Read the model definition and answer for the solid it produces. Units are mm, in the model's axes. Face numbers are marked on the shaded views. A direction names the side the tool comes from. Give positions to 0.01 mm unless a question says otherwise; leave off trailing zeros. Loops run counter-clockwise (first coordinate to the right, second up) from the corner with the lowest first, then second, coordinate; pieces in that order, holes last. Notation, with made-up numbers: (0.5, 80) - (5.5, 80) arc R27 ccw to (5.5, 110) - close; hole circle Ø4 at (74.5, 69). An arc over 180 degrees is marked (long way). Write item = value, one per line.
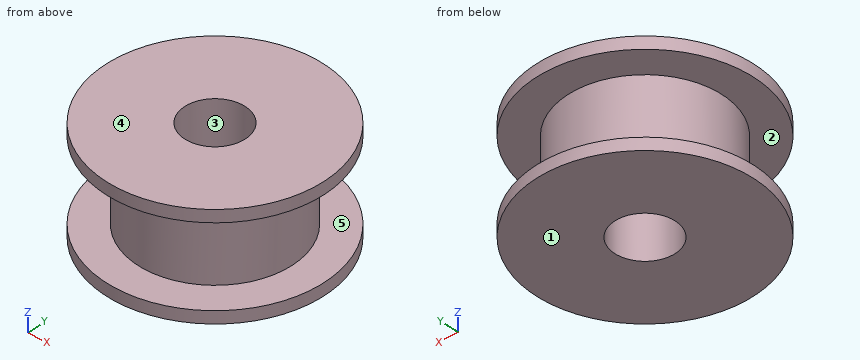
Autodesk Inventor part; units mm, degrees
ref_plane "YZ Plane" through (0, 0, 0) normal (1, 0, 0) x (0, 1, 0)
ref_plane "XZ Plane" through (0, 0, 0) normal (0, 1, 0) x (-1, 0, 0)
ref_plane "XY Plane" through (0, 0, 0) normal (0, 0, 1) x (1, 0, 0)
sketch "Sketch1" plane through (0, 0, 0) normal (0, 0, 1) x (1, 0, 0)
  circle A0 centre (0, 0) radius 6.3662
  dimension "d0" = 12.7324
extrude "Extrusion1" add sketch "Sketch1" along normal blind 8.6
sketch "Sketch2" plane through (0, 0, 8.6) normal (0, 0, 1) x (1, 0, 0)
  circle A0 centre (0, 0) radius 6.3662
  circle A1 centre (0, 0) radius 9
  dimension "d5" = 18
extrude "Extrusion2" add sketch "Sketch2" against normal blind 1
sketch "Sketch3" plane through (0, 0, 0) normal (0, 0, -1) x (-1, 0, 0)
  circle A0 centre (0, 0) radius 6.3662
  circle A1 centre (0, 0) radius 6.3662
  circle A2 centre (0, 0) radius 9
extrude "Extrusion3" add sketch "Sketch3" against normal blind 1
sketch "Sketch4" plane through (0, 0, 0) normal (0, 0, -1) x (-1, 0, 0)
  circle A0 centre (0, 0) radius 9
  circle A1 centre (0, 0) radius 2.5
  dimension "d11" = 5
extrude "Extrusion4" cut sketch "Sketch4" against normal through all contours A1
properties part number "idler"
1) A tool of negligible diameter and unlimited length cuts with its end or side. For the marked faces 1 and 2, from which of +Z, -Z, +X, -X, +Y, -Y can it reach the whole face along a straight path? Write none if from no direction.
Output:
face_1 = -Z, +X, -X, +Y, -Y
face_2 = none
2) The mould has two halves that part along Z. Classify the marked faces 3, 4 and 5: pulls with the +Z half, pulls with the -Z half, needs draft (parallel to the pull), parting line crosses it, or undercut.
Output:
face_3 = needs draft
face_4 = pulls with the +Z half
face_5 = undercut
3) A cutting plane is placed at C-C on y = -3.75. Determine the outline of the cut face in (x, z).
Output:
outline = (-8.18, 0) - (8.18, 0) - (8.18, 1) - (5.14, 1) - (5.14, 7.6) - (8.18, 7.6) - (8.18, 8.6) - (-8.18, 8.6) - (-8.18, 7.6) - (-5.14, 7.6) - (-5.14, 1) - (-8.18, 1) - close
4) A cutting plane is placed at D-D on z = 4. Determine the outline of the cut face in (x, y), then the cut area to 3 significant figures.
Output:
outline = circle Ø12.73 at (0, 0); hole circle Ø5 at (0, 0)
area = 108 mm²
5) A cutting plane is placed at A-A on y = 0. Determine the outline of the cut face in (x, z).
Output:
outline = (-9, 0) - (-2.5, 0) - (-2.5, 8.6) - (-9, 8.6) - (-9, 7.6) - (-6.37, 7.6) - (-6.37, 1) - (-9, 1) - close; (2.5, 0) - (9, 0) - (9, 1) - (6.37, 1) - (6.37, 7.6) - (9, 7.6) - (9, 8.6) - (2.5, 8.6) - close
6) Find the intervals of material crossed by probe 1 along Z at (x, y) = (-6.5, 4.5); probe 2 along Y at (x, z) = (0, 2); probe 3 along Y at (x, z) = (-1, 6), in increasing order.
Output:
probe_1 = 0 to 1, 7.6 to 8.6
probe_2 = -6.37 to -2.5, 2.5 to 6.37
probe_3 = -6.29 to -2.29, 2.29 to 6.29
7) Each of these flat-tipped pins is pushed along its axis until it touches: P1, Ø5, axis at y = -4, z = 6, coming from the +X side; P2, Ø1, axis at y = -3.5, z = 6, coming from the +X side (3 decimals); P3, Ø1.5, axis at x = 6, z = 7.5, coming from the -Y side. Where does it stop, or does it pass through?
Output:
P1 = 8.76
P2 = 5.615
P3 = -7.31
